from build123d import *

# Parameters (mm, degrees)
BOSS_EXTRUDE1_DEPTH         = 1.5875
F_1_4_0_25_DIAMETER_HOLE1_D = 6.35


with BuildPart() as part:
    # Sketch1 → Boss-Extrude1 (new body)
    with BuildSketch(Plane.XY):
        Polygon((0, 0), (53.18125, 0), (421.48125, 276.225), (451.96125, 235.585), (87.047916667, -38.1), (38.1, -38.1), align=None)
    extrude(amount=BOSS_EXTRUDE1_DEPTH)

    # 1/4 (0.25) Diameter Hole1 (through all)
    with Locations(Plane.XY.offset(1.5875)):
        with Locations((428.77096872, 234.06728904), (271.29096872, 115.95728904), (113.81096872, -2.15271096)):
            Hole(F_1_4_0_25_DIAMETER_HOLE1_D / 2)


solid = part.part
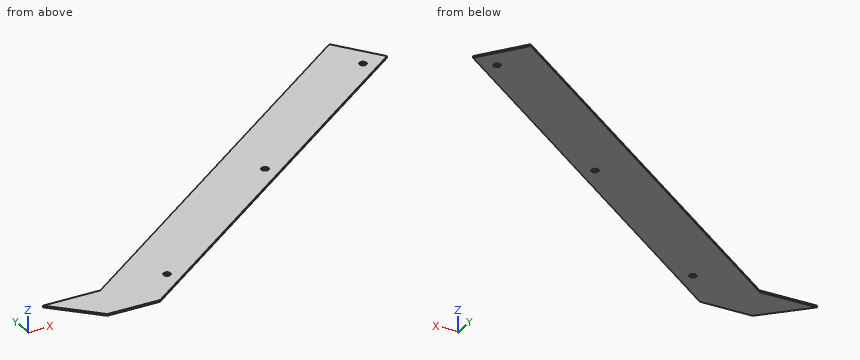
Build history of the part. All positions in model axes, mm. Round coordinates to 2 decimals unless told otherwise and drop trailing zeros. Write each loop counter-clockwise with the first axis right and the second up, starting at its lowest first coordinate (ties: lowest second). Pieces come first, ordered by that corner, then holes. Notation, with made-up numbers: M -5,-5 L 41,-5 A18 ccw 41,10 Z; hole C -20,-26.5 d3. An arc over 180 degrees is marked long. Use CSV: the item, a comma, the result in double quotes.
1. Wall check: probe 1 along Y at (x, z) = (44.5, 0.5); probe 2 along Y at (x, z) = (357.5, 1.15); probe 3 along X at (y, z) = (55, 0.95). Give the ranges that are in metal, low to high. Write a range as from..to.
Reply:
probe 1,"y = -38.1..0"
probe 2,"y = 164.74..228.24"
probe 3,"x = 126.51..211.18"
2. Saw through at A-A (z = 1.3). Give the cut face in (x, y) (3 decimals).
Reply:
outline,"M 0,0 L 38.1,-38.1 L 87.048,-38.1 L 451.961,235.585 L 421.481,276.225 L 53.181,0 Z; hole C 113.811,-2.153 d6.35; hole C 271.291,115.957 d6.35; hole C 428.771,234.067 d6.35"
3. Saw through at B-B (y = 97.5). Give the cut face in (x, z).
Reply:
outline,"M 183.18,0 L 267.85,0 L 267.85,1.59 L 183.18,1.59 Z"
4. Flat gauge pins, fed straight in: pin 1 (0.8 mm diameter, centred on x = 34, z = 1, fed in from +Y); pin 2 (8.5 mm diameter, centred on x = 113.81, y = -2.15, fed in from +Z). Where does each tip first touch, or does it go through?
Reply:
pin 1,"stops at y = 0"
pin 2,"stops at z = 1.59"
5. Saw through at C-C (x = 149). Give the cut face in (y, z), plus the area to 3 significant figures.
Reply:
outline,"M 8.36,0 L 71.86,0 L 71.86,1.59 L 8.36,1.59 Z"
area,"101 mm²"
